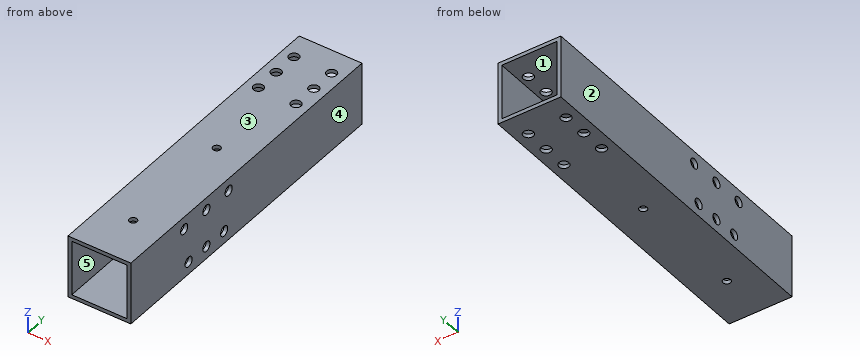
from build123d import *

# Parameters (mm, degrees)
BOSS_EXTRUDE1_DEPTH      = 65
BOSS_EXTRUDE1_DEPTH_BACK = 65
SKETCH3_W                = 25
SKETCH3_H                = 25
SKETCH3_W_2              = 22
SKETCH3_H_2              = 22
SKETCH5_R                = 1.5
CUT_EXTRUDE2_DEPTH       = 25
SKETCH6_R                = 2
CUT_EXTRUDE3_DEPTH       = 25
SKETCH7_R                = 2
CUT_EXTRUDE4_DEPTH       = 25


with BuildPart() as part:
    # Sketch3 → Boss-Extrude1 (new, two sides: drawn at the far end of the back side and taken through both)
    with BuildSketch(Plane(origin=(0, 0, 0), x_dir=(1, 0, 0), z_dir=(0, 1, 0)).offset(-BOSS_EXTRUDE1_DEPTH_BACK)):
        Rectangle(SKETCH3_W, SKETCH3_H)
        Rectangle(SKETCH3_W_2, SKETCH3_H_2, mode=Mode.SUBTRACT)
    extrude(amount=BOSS_EXTRUDE1_DEPTH + BOSS_EXTRUDE1_DEPTH_BACK)

    # Sketch5 → Cut-Extrude2 (cut)
    with BuildSketch(Plane(origin=(0, 0, -12.5), x_dir=(-1, 0, 0), z_dir=(0, 0, -1))):
        with Locations((0, -46)):
            Circle(SKETCH5_R)
        with Locations((0, 1)):
            Circle(SKETCH5_R)
    extrude(amount=-CUT_EXTRUDE2_DEPTH, mode=Mode.SUBTRACT)

    # Sketch6 → Cut-Extrude3 (cut)
    with BuildSketch(Plane(origin=(12.5, 0, 0), x_dir=(0, 0, -1), z_dir=(1, 0, 0))):
        with Locations((7.5, -32.5)):
            Circle(SKETCH6_R)
        with Locations((7.5, -12.5)):
            Circle(SKETCH6_R)
        with Locations((-7.5, -35)):
            Circle(SKETCH6_R)
        with Locations((-7.5, -10)):
            Circle(SKETCH6_R)
        with Locations((7.5, -22.5)):
            Circle(SKETCH6_R)
        with Locations((-7.5, -22.5)):
            Circle(SKETCH6_R)
    extrude(amount=-CUT_EXTRUDE3_DEPTH, mode=Mode.SUBTRACT)

    # Sketch7 → Cut-Extrude4 (cut)
    with BuildSketch(Plane(origin=(0, 0, -12.5), x_dir=(-1, 0, 0), z_dir=(0, 0, -1))):
        with Locations((7.5, 55)):
            Circle(SKETCH7_R)
        with Locations((7.5, 45)):
            Circle(SKETCH7_R)
        with Locations((-7.5, 55)):
            Circle(SKETCH7_R)
        with Locations((-7.5, 45)):
            Circle(SKETCH7_R)
        with Locations((-7.5, 35)):
            Circle(SKETCH7_R)
        with Locations((7.5, 35)):
            Circle(SKETCH7_R)
    extrude(amount=-CUT_EXTRUDE4_DEPTH, mode=Mode.SUBTRACT)


solid = part.part
Build history of the part. All positions in model axes, mm. Face numbers are marked on the shaded views. A direction names the side the tool comes from. Coordinates: 2 decimals unless noted, no trailing zeros. Order: outer loops, then holes, each group sorted by start corner. A loop starts at its lowest first (then second) coordinate and runs counter-clockwise, first axis right, second up. Notation, with made-up numbers: (-22.5, -2) - (-1.5, -2) arc R10 cw to (-1.5, 13) - close; hole circle Ø6 at (46, 81). An arc over 180 degrees is marked (long way). Put each result on its own line as item: value.
1. Saw through at B-B (y = -22.5). Write the cut outline in (x, z).
Answer sheet:
outline: (-12.5, -12.5) - (12.5, -12.5) - (12.5, -9.5) - (11, -9.5) - (11, -11) - (-11, -11) - (-11, -9.5) - (-12.5, -9.5) - close; (-12.5, -5.5) - (-11, -5.5) - (-11, 5.5) - (-12.5, 5.5) - close; (-12.5, 9.5) - (-11, 9.5) - (-11, 11) - (11, 11) - (11, 9.5) - (12.5, 9.5) - (12.5, 12.5) - (-12.5, 12.5) - close; (11, -5.5) - (12.5, -5.5) - (12.5, 5.5) - (11, 5.5) - close
2. Pull direction X, two halves, no side cores. Call the marked faces 3, 4 and 5: pulls with the +X half, pulls with the -X half, needs draft (parallel to the pull), parting line crosses it, or undercut.
Answer sheet:
face 3: needs draft
face 4: pulls with the +X half
face 5: undercut
3. Probe line 1 along Y through (x, z) = (7.5, -11.35); line 2 along Y through (x, z) = (-11.4, -7.5); line 3 along Y through (x, z) = (0, 11.45). List the from-to ranges inside material, lowest first. Write a range as [from, to].
Answer sheet:
line 1: y = [-65, 33], [37, 43], [47, 53], [57, 65]
line 2: y = [-65, -34.5], [-30.5, -24.5], [-20.5, -14.5], [-10.5, 65]
line 3: y = [-65, -47.5], [-44.5, -0.5], [2.5, 65]
4. Saw through at C-C (x = -7.5). Give the number of separate pieces and of enclosed holes in the cut face, and give its area (3 significant figures).
Answer sheet:
separate pieces: 8
enclosed holes: 0
area: 354 mm^2
5. Saw through at A-A (z = 0). Write the cut outline in (x, y), and give its area (3 significant figures).
Answer sheet:
outline: (-12.5, -65) - (-11, -65) - (-11, 65) - (-12.5, 65) - close; (11, -65) - (12.5, -65) - (12.5, 65) - (11, 65) - close
area: 390 mm^2
6. Saw through at D-D (x = 0). Write the cut outline in (y, z), and give its area (3 significant figures).
Answer sheet:
outline: (-65, -12.5) - (-47.5, -12.5) - (-47.5, -11) - (-65, -11) - close; (-65, 11) - (-47.5, 11) - (-47.5, 12.5) - (-65, 12.5) - close; (-44.5, -12.5) - (-0.5, -12.5) - (-0.5, -11) - (-44.5, -11) - close; (-44.5, 11) - (-0.5, 11) - (-0.5, 12.5) - (-44.5, 12.5) - close; (2.5, -12.5) - (65, -12.5) - (65, -11) - (2.5, -11) - close; (2.5, 11) - (65, 11) - (65, 12.5) - (2.5, 12.5) - close
area: 372 mm^2
7. Tool access for the marked faces 1 and 2: list every direction of +Z, -Z, +X, -X, +Y, -Y with a clear straight run to the whole face (end or side of a thin tool).
Answer sheet:
face 1: +Y, -Y
face 2: +Z, -Z, -X, +Y, -Y
